Design review of the part shown in the three views and the two pictorial views. Dimensions are in mm from the part's minimum x, y and z. A direction names the side the tool comes from. Give positions to 0.01 mm unless a question says otherwise; leave off trailing zeros. Order: outer loops, then holes, each group sorted by start corner. A loop starts at its lowest first (then second) coordinate and runs counter-clockwise, first axis right, second up. Notation, with made-up numbers: (82, 31.25) -> (141, 31.25) arc R16 ccw to (141, 49.25) -> close; hole circle Ø7 at (34, 11.5). An arc over 180 degrees is marked (long way). Answer in a Markdown table with one row per item. Add a question column.
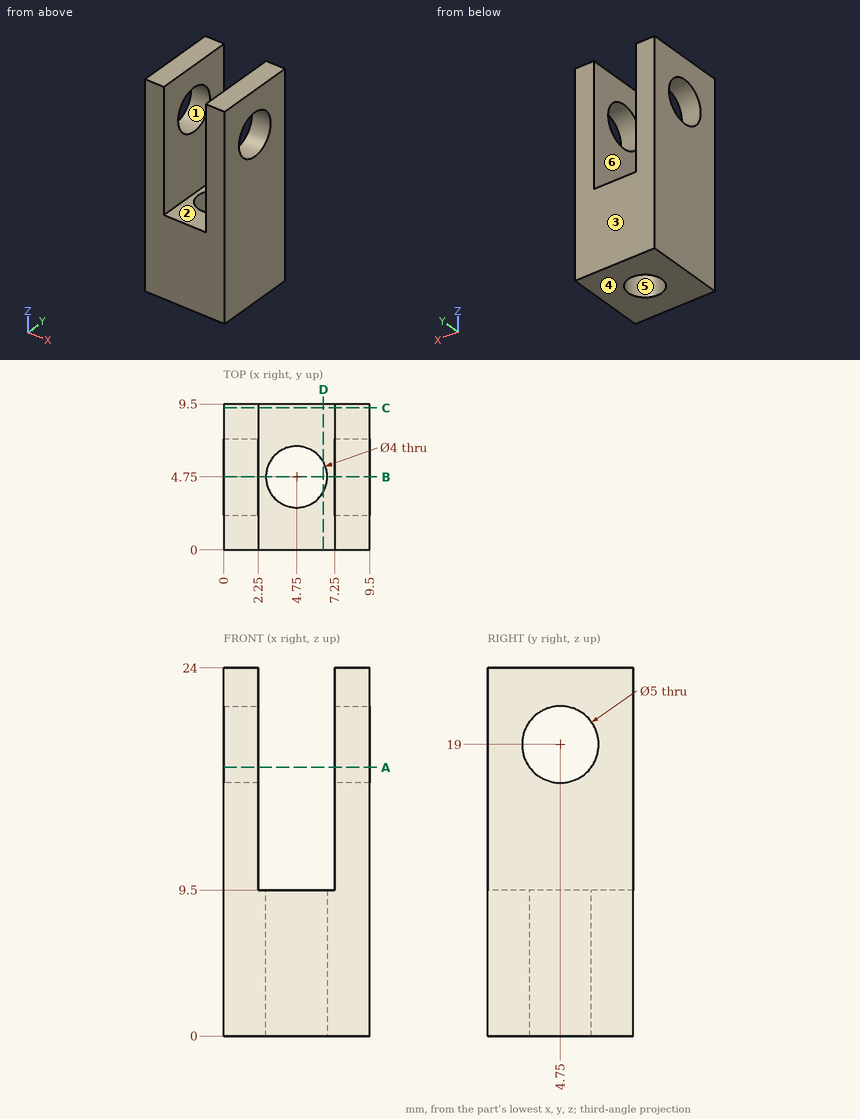
1) Add section A-A, the plane z = 17.5. Write out the cut boundary in (x, y).
2) Add section B-B, the plane y = 4.75. Write out the cut boundary in (x, z).
3) For L1, parallel to Y at x = 0.7, z = 19; L2, parallel to Y at x = 4.75, z = 7.25, list the stretches that pass through material, from the lowest coordinate up.
4) Machinability: for the marked faces 5 and 6, which of the approach directions +Z, -Z, +X, -X, +Y, -Y give a long, thin tool a straight path to every point of the face, cutting with its end or side? Answer none if there is none.
5) Add section C-C, the plane y = 9.25. Write out the cut boundary in (x, z).
6) Add section D-D, the plane x = 6.5. Write out the cut boundary in (y, z), and give its area (3 significant figures).
7) Clearance check with flat-ended pins moving along their axes: P1, Ø4, axis at y = 4.75, z = 19, coming from the -X side; P2, Ø4.5, axis at x = 4.75, y = 4.75, coming from the +Z side. State where each tip first meets the part, or that it passes through.
8) Mouldability with a two-part tool opening along Z and no side actions: class the marked faces 1, 2, 3 and 4 as +Z half, -Z half, draft (parallel to the pull), parting line (faces both ways), or undercut.
Verdict:
| question | item | result |
|---|---|---|
| 1 | outline | (0, 0) -> (2.25, 0) -> (2.25, 2.75) -> (0, 2.75) -> close; (0, 6.75) -> (2.25, 6.75) -> (2.25, 9.5) -> (0, 9.5) -> close; (7.25, 0) -> (9.5, 0) -> (9.5, 2.75) -> (7.25, 2.75) -> close; (7.25, 6.75) -> (9.5, 6.75) -> (9.5, 9.5) -> (7.25, 9.5) -> close |
| 2 | outline | (0, 0) -> (2.75, 0) -> (2.75, 9.5) -> (2.25, 9.5) -> (2.25, 16.5) -> (0, 16.5) -> close; (0, 21.5) -> (2.25, 21.5) -> (2.25, 24) -> (0, 24) -> close; (6.75, 0) -> (9.5, 0) -> (9.5, 16.5) -> (7.25, 16.5) -> (7.25, 9.5) -> (6.75, 9.5) -> close; (7.25, 21.5) -> (9.5, 21.5) -> (9.5, 24) -> (7.25, 24) -> close |
| 3 | L1 | y = 0 to 2.25, 7.25 to 9.5 |
| 3 | L2 | y = 0 to 2.75, 6.75 to 9.5 |
| 4 | face 5 | +Z, -Z |
| 4 | face 6 | +Z, +Y, -Y |
| 5 | outline | (0, 0) -> (9.5, 0) -> (9.5, 24) -> (7.25, 24) -> (7.25, 9.5) -> (2.25, 9.5) -> (2.25, 24) -> (0, 24) -> close |
| 6 | outline | (0, 0) -> (3.78, 0) -> (3.78, 9.5) -> (0, 9.5) -> close; (5.72, 0) -> (9.5, 0) -> (9.5, 9.5) -> (5.72, 9.5) -> close |
| 6 | area | 71.9 mm2 |
| 7 | P1 | passes through |
| 7 | P2 | stops at z = 9.5 |
| 8 | face 1 | undercut |
| 8 | face 2 | +Z half |
| 8 | face 3 | draft |
| 8 | face 4 | -Z half |
